The figure shows three views and two pictorial views of one solid part (mm, origin at its lowest corner). Answer the questions. A direction names the side the tool comes from. Round coordinates to 2 decimals unless told otherwise and drop trailing zeros. Order: outer loops, then holes, each group sorted by start corner. A loop starts at its lowest first (then second) coordinate and runs counter-clockwise, first axis right, second up. Notation, with made-up numbers: (59, -9) - (102, -9) arc R9 ccw to (102, 3) - close; hole circle Ø8 at (70.25, 65). An arc over 180 degrees is marked (long way). Answer in a Markdown table with one row per item.
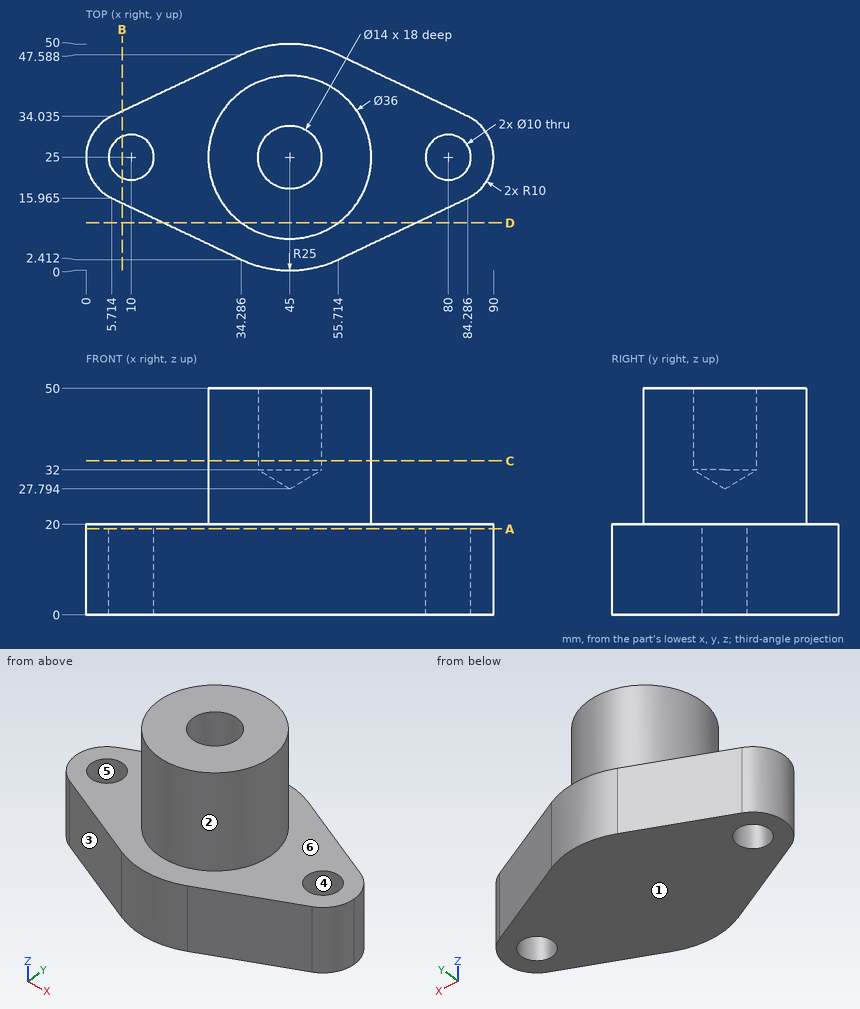
1) Find section D-D, the plane y = 10.5. Give the vertices of the cut face in (x, z) (1 decimal).
Filled in:
| item | result |
|---|---|
| outline | (17.2, 0) - (72.8, 0) - (72.8, 20) - (55.7, 20) - (55.7, 50) - (34.3, 50) - (34.3, 20) - (17.2, 20) - close |
2) The mould has two halves that part along Y. Classify the marked faces 3, 4, 5 and 6: released by +Y, released by -Y, zero draft, split by the parting line, or undercut.
Filled in:
| item | result |
|---|---|
| face 3 | released by -Y |
| face 4 | undercut |
| face 5 | undercut |
| face 6 | zero draft |
3) Find section A-A, the plane z = 19. Give the vertices of the cut face in (x, y) (1 decimal), then the cut area to 3 significant figures.
Filled in:
| item | result |
|---|---|
| outline | (5.7, 16) - (34.3, 2.4) arc R25 ccw to (55.7, 2.4) - (84.3, 16) arc R10 ccw to (84.3, 34) - (55.7, 47.6) arc R25 ccw to (34.3, 47.6) - (5.7, 34) arc R10 ccw to start; hole circle Ø10 at (10, 25); hole circle Ø10 at (80, 25) |
| area | 2,840 mm^2 |
4) Find the intervals of material crossed by probe 1 along X at (y, z) = (25, 5.25); probe 2 along Y at (x, z) = (45, 43); probe 3 along Z at (x, y) = (47.5, 5), in increasing order. Write a range as from..to.
Filled in:
| item | result |
|---|---|
| probe 1 | x = 0..5, 15..75, 85..90 |
| probe 2 | y = 7..18, 32..43 |
| probe 3 | z = 0..20 |
5) Which of the six approach directions +Z, -Z, +X, -X, +Y, -Y give full straight-line access (tool end or side, diameter ignored) to the marked faces 1 and 2?
Filled in:
| item | result |
|---|---|
| face 1 | -Z, +X, -X, +Y, -Y |
| face 2 | +Z |
6) Find section B-B, the plane x = 8. Give the vertices of the cut face in (y, z).
Filled in:
| item | result |
|---|---|
| outline | (14.88, 0) - (20.42, 0) - (20.42, 20) - (14.88, 20) - close; (29.58, 0) - (35.12, 0) - (35.12, 20) - (29.58, 20) - close |
7) Find section C-C, the plane z = 34. Give the vertices of the cut face in (x, y).
Filled in:
| item | result |
|---|---|
| outline | circle Ø36 at (45, 25); hole circle Ø14 at (45, 25) |
8) Each of these flat-tipped pins is pushed along its axis until it touches: pin 1 (2 mm diameter, centred on y = 15, z = 27, fed in from +X); pin 2 (12 mm diameter, centred on y = 42, z = 33, fed in from +X); pin 3 (8 mm diameter, centred on x = 67.5, z = 21.5, fed in from +Y); pin 4 (18 mm diameter, centred on x = 45, y = 25, fed in from +Z). Where does it stop, or does it pass through?
Filled in:
| item | result |
|---|---|
| pin 1 | stops at x = 60.59 |
| pin 2 | stops at x = 59.25 |
| pin 3 | stops at y = 43.76 |
| pin 4 | stops at z = 50 |
